Part print with two shaded views. Sizes in mm from the minimum x, y, z corner. Round coordinates to 2 decimals unless told otherwise and drop trailing zeros. Loops run counter-clockwise (first coordinate to the right, second up) from the corner with the lowest first, then second, coordinate; pieces in that order, holes last. Notation, with made-up numbers: (69.5, 80.25) -> (94.5, 80.25) arc R8 cw to (94.5, 91.25) -> close; hole circle Ø7 at (0, 2). An arc over 180 degrees is marked (long way). Use a Markdown table: item, result. Add a question column.
Item 1: Cut at D-D, the plane y = 12. List the corners of the cut face in (x, z), plus the area to 3 significant figures.
Item 2: Flat gauge pins, fed straight in: pin 1 (4.5 mm diameter, centred on x = 28.5, y = 16, fed in from +Z); pin 2 (1 mm diameter, centred on y = 32, z = 91, fed in from -X); pin 3 (4 mm diameter, centred on x = 26, y = 22, fed in from +Z). Where does each tip first touch, or does it go through?
Item 3: Probe line 1 (Y direction, x = 28.4, z = 92.75); line 2 (Z direction, x = 21, y = 45.5); line 3 (Z direction, x = 24, y = 46.5). List the from-to ranges inside material, lowest first. Write a range as [from, to].
Item 4: Cut at B-B, the plane z = 36. List the corners of the cut face in (x, y).
Item 5: Cut at A-A, the plane y = 35. List the corners of the cut face in (x, z), plus the area to 3 significant figures.
Item 6: Cut at C-C, the plane x = 35.4. List the corners of the cut face in (y, z), plus the area to 3 significant figures.
Item 7: Two-plate mould, pull along Z, no slides. Class the marked faces 1, 2 and 3: pulls with the +Z half, pulls with the -Z half, needs draft (parallel to the pull), parting line crosses it, or undercut.
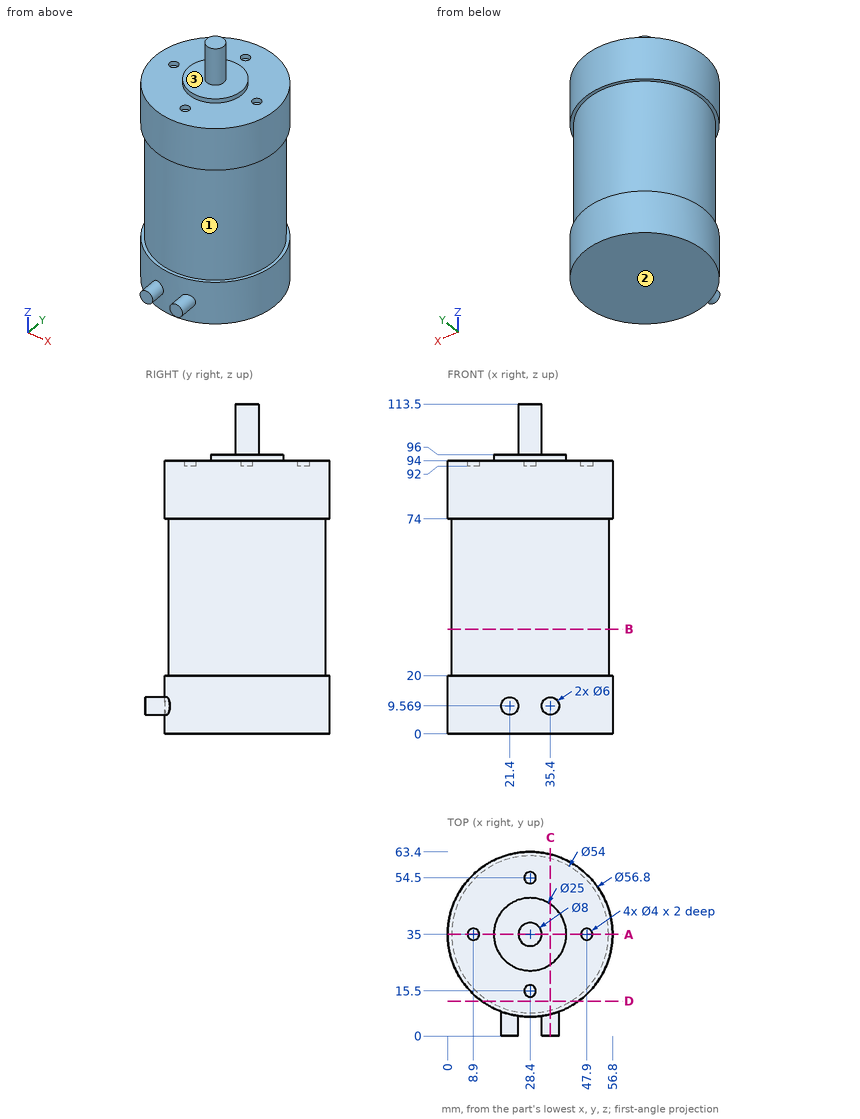
A:
| question | item | result |
|---|---|---|
| 1 | outline | (11.74, 0) -> (45.06, 0) -> (45.06, 20) -> (42.54, 20) -> (42.54, 74) -> (45.06, 74) -> (45.06, 94) -> (11.74, 94) -> (11.74, 74) -> (14.26, 74) -> (14.26, 20) -> (11.74, 20) -> close |
| 1 | area | 2,860 mm^2 |
| 2 | pin 1 | stops at z = 94 |
| 2 | pin 2 | stops at x = 0.11 |
| 2 | pin 3 | stops at z = 96 |
| 3 | line 1 | y = [6.6, 13.5], [17.5, 52.5], [56.5, 63.4] |
| 3 | line 2 | z = [0, 94] |
| 3 | line 3 | z = [0, 96] |
| 4 | outline | circle Ø54 at (28.4, 35) |
| 5 | outline | (0, 0) -> (56.8, 0) -> (56.8, 20) -> (55.4, 20) -> (55.4, 74) -> (56.8, 74) -> (56.8, 94) -> (49.9, 94) -> (49.9, 92) -> (45.9, 92) -> (45.9, 94) -> (40.9, 94) -> (40.9, 96) -> (32.4, 96) -> (32.4, 113.5) -> (24.4, 113.5) -> (24.4, 96) -> (15.9, 96) -> (15.9, 94) -> (10.9, 94) -> (10.9, 92) -> (6.9, 92) -> (6.9, 94) -> (0, 94) -> (0, 74) -> (1.4, 74) -> (1.4, 20) -> (0, 20) -> close |
| 5 | area | 5,360 mm^2 |
| 6 | outline | (0, 6.57) -> (7.48, 6.57) -> (7.48, 0) -> (62.52, 0) -> (62.52, 20) -> (61.08, 20) -> (61.08, 74) -> (62.52, 74) -> (62.52, 94) -> (45.36, 94) -> (45.36, 96) -> (24.64, 96) -> (24.64, 94) -> (7.48, 94) -> (7.48, 74) -> (8.92, 74) -> (8.92, 20) -> (7.48, 20) -> (7.48, 12.57) -> (0, 12.57) -> close |
| 6 | area | 5,100 mm^2 |
| 7 | face 1 | undercut |
| 7 | face 2 | pulls with the -Z half |
| 7 | face 3 | pulls with the +Z half |
